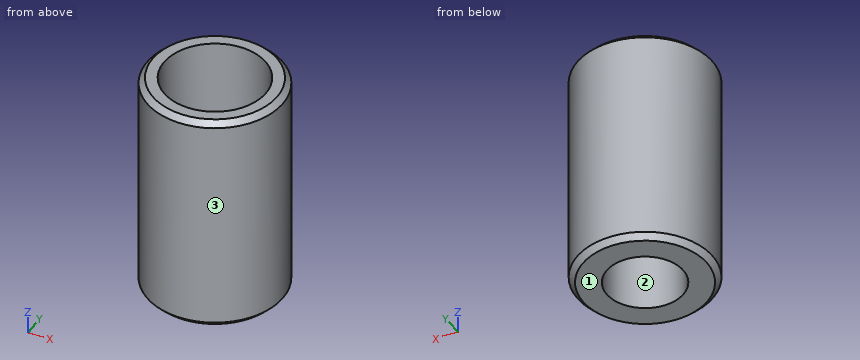
Autodesk Inventor part; units mm, degrees
ref_plane "YZ Plane" through (0, 0, 0) normal (1, 0, 0) x (0, 1, 0)
ref_plane "XZ Plane" through (0, 0, 0) normal (0, 1, 0) x (-1, 0, 0)
ref_plane "XY Plane" through (0, 0, 0) normal (0, 0, 1) x (1, 0, 0)
sketch "Sketch1" plane through (0, 0, 0) normal (0, 0, 1) x (1, 0, 0)
  circle A0 centre (0, 0) radius 38.1
  dimension "d0" = 76.2
extrude "Extrusion1" add sketch "Sketch1" along normal blind 127
chamfer "Chamfer1" distance 3.175 angle 45 2 edges at (-38.1, 0, 0) (-38.1, 0, 127)
sketch "Sketch2" plane through (0, 0, 127) normal (0, 0, 1) x (1, 0, 0)
  point P0 (0, 0)
hole "Hole1" at (0, 0, 127) direction (0, 0, -1) diameter 43.18 end through all counterbore diameter 57.15 counterbore depth 63.5
properties part number "Coupler" material "Steel, Mild"
Part model, mm, in its own coordinate system. Face numbers are marked on the shaded views. Round coordinates to 2 decimals unless told otherwise and drop trailing zeros. Order: outer loops, then holes, each group sorted by start corner. A loop starts at its lowest first (then second) coordinate and runs counter-clockwise, first axis right, second up. Notation, with made-up numbers: M 52.5,65.5 L 66.5,65.5 A10 ccw 66.5,80.5 Z; hole C 81,-9 d7. An arc over 180 degrees is marked long. Answer in a Markdown table with one row per item. Add a question column.
Q1. Cut at C-C on z = 65. Give the cut face in (x, y) (3 decimals).
Q2. Cut at A-A on y = 0. Give the cut face in (x, z) (3 decimals).
Q3. Pin check, flat tips, straight feed: pin 1 (1.5 mm diameter, centred on x = 17.5, z = 76, fed in from -Y); pin 2 (5 mm diameter, centred on x = -29, z = 37.5, fed in from +Y); pin 3 (1 mm diameter, centred on y = 17.5, z = 37.5, fed in from -X). Stop position of each tip, or through.
Q4. Mould opens along X. For the marked faces 1, 2 and 3 say: +X half, -X half, draft (parallel to the pull), parting line (faces both ways), or undercut.
Q5. Wall check: L1, parallel to Y at x = 0, z = 107 (3 decimals); L2, parallel to Y at x = 0, z = 44.5; L3, parallel to Z at x = 10, y = -24. Give the ranges that are in metal, low to high. Write a range as from..to.
Q6. Cut at D-D on z = 12.5. Give the cut face in (x, y).
Established:
| question | item | result |
|---|---|---|
| 1 | outline | C 0,0 d76.2; hole C 0,0 d57.15 |
| 2 | outline | M -38.1,3.175 L -34.925,0 L -21.59,0 L -21.59,63.5 L -28.575,63.5 L -28.575,127 L -34.925,127 L -38.1,123.825 Z; M 21.59,0 L 34.925,0 L 38.1,3.175 L 38.1,123.825 L 34.925,127 L 28.575,127 L 28.575,63.5 L 21.59,63.5 Z |
| 3 | pin 1 | stops at y = -34.22 |
| 3 | pin 2 | stops at y = 27.37 |
| 3 | pin 3 | stops at x = -34.1 |
| 4 | face 1 | draft |
| 4 | face 2 | undercut |
| 4 | face 3 | parting line |
| 5 | L1 | y = -38.1..-28.575, 28.575..38.1 |
| 5 | L2 | y = -38.1..-21.59, 21.59..38.1 |
| 5 | L3 | z = 0..63.5 |
| 6 | outline | C 0,0 d76.2; hole C 0,0 d43.18 |
